Check sheet for the drawn part. Datum: minimum x, y, z corner. Units: mm. A direction names the side the tool comes from. Give positions to 0.01 mm unless a question says otherwise; leave off trailing zeros. Order: outer loops, then holes, each group sorted by start corner. A loop starts at its lowest first (then second) coordinate and runs counter-clockwise, first axis right, second up. Notation, with made-up numbers: (12.25, 88) -> (63.25, 88) arc R21 cw to (63.25, 93) -> close; hole circle Ø6 at (87, 36.25). An arc over 180 degrees is marked (long way). Return JSON: item names as keys, results as strings. Group by question number.
(1) Cross-section at B-B on z = 4. Enter the section's corners in (x, y).
(2) Thickness scan on line 1 along X through (y, z) = (1.35, 4); line 2 along X through (y, z) = (14, 3.75). Record the ranges inside material, lowest first.
(3) Cross-section at D-D on z = 7. Enter the section's corners in (x, y).
(4) Tool access check on the marked faces 1 and 2. Record the directions out of +Z, -Z, +X, -X, +Y, -Y that give a thin tool (end or side, any length) a straight path to the whole face; none if there is none.
(5) Depth check by flat-ended pin: pin 1 Ø4 at (y, z) = (8, 2) entering from +X; pin 2 Ø2 at (x, z) = (1.5, 5) entering from -Y; pin 3 Ø3 at (x, z) = (8, 5.5) entering from +Y. Enter the tip coordinate at first touch or a pass-through.
(6) Cross-section at A-A on x = 8.5. Enter the section's corners in (y, z), then the cut area to 3 significant figures.
(7) Release check for a two-part mould opening along Z. For the marked faces 3, 4, 5 and 6 record: pulls with the +Z half, pulls with the -Z half, needs draft (parallel to the pull), parting line crosses it, or undercut.
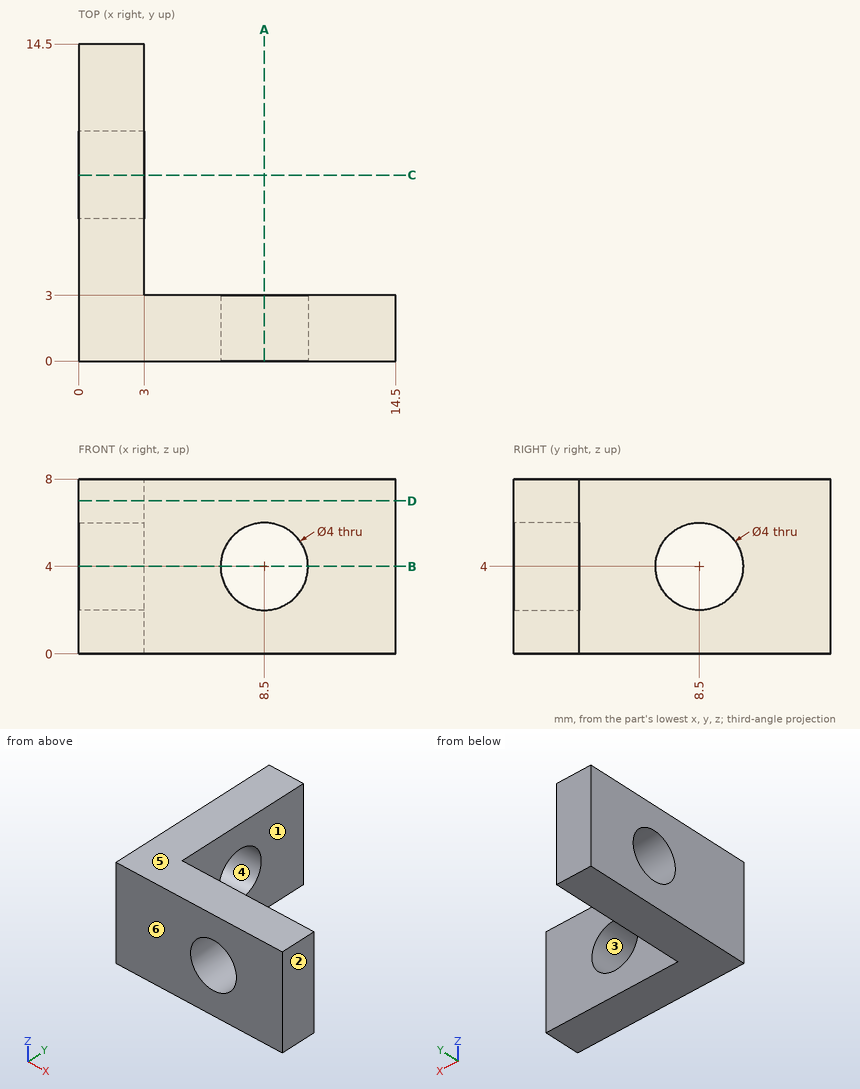
Verdict:
{
 "1": {"outline": "(0, 0) -> (6.5, 0) -> (6.5, 3) -> (3, 3) -> (3, 6.5) -> (0, 6.5) -> close; (0, 10.5) -> (3, 10.5) -> (3, 14.5) -> (0, 14.5) -> close; (10.5, 0) -> (14.5, 0) -> (14.5, 3) -> (10.5, 3) -> close"},
 "2": {"line 1": "0 to 6.5, 10.5 to 14.5", "line 2": "0 to 3"},
 "3": {"outline": "(0, 0) -> (14.5, 0) -> (14.5, 3) -> (3, 3) -> (3, 14.5) -> (0, 14.5) -> close"},
 "4": {"face 1": "+Z, -Z, +X, +Y", "face 2": "+Z, -Z, +X, +Y, -Y"},
 "5": {"pin 1": "x = 3", "pin 2": "y = 0", "pin 3": "y = 3"},
 "6": {"outline": "(0, 0) -> (3, 0) -> (3, 2) -> (0, 2) -> close; (0, 6) -> (3, 6) -> (3, 8) -> (0, 8) -> close", "area": "12.0 mm²"},
 "7": {"face 3": "undercut", "face 4": "undercut", "face 5": "pulls with the +Z half", "face 6": "needs draft"}
}
